Check sheet for the modelled part. Datum: model origin and axes. Units: mm. Round coordinates to 2 decimals unless told otherwise and drop trailing zeros. Loops run counter-clockwise (first coordinate to the right, second up) from the corner with the lowest first, then second, coordinate; pieces in that order, holes last. Notation, with made-up numbers: (-0.75, 5) - (40.25, 5) arc R29 cw to (40.25, 42) - close; hole circle Ø6 at (42.5, 43.25). An arc over 180 degrees is marked (long way). Put each result on its own line as item: value. Start each with the question number.
Item 1: Section check D-D, the plane x = 32. Record the cut outline in (y, z), and give its area (3 significant figures).
Item 2: Section check B-B, the plane y = 12.2. Record the cut outline in (x, z).
Item 3: Draft check along X on faces 1 (the flat face through (1, 10, -1)), 2 (the cylindrical face through (-0.1, 11.52, -13.24)). Enter one of: pulls with the +X half, pulls with the -X half, needs draft (parallel to the pull), parting line crosses it, or undercut.
Item 4: Section check C-C, the plane z = -43.5. Record the cut outline in (x, y), and give its area (3 significant figures).
Item 5: Section check A-A, the plane x = 11. Record the cut outline in (y, z).
Item 6: Gauge pin test, flat ends, axial feed: pin 1 Ø1 at (x, y) = (-33.5, 11.5) entering from +Z; pin 2 Ø0.9 at (y, z) = (12, -78.5) entering from +X; pin 3 Ø1.5 at (x, y) = (-58, 11.5) entering from -Z. Record the tip position at first contact, or that the pin passes through.
Item 7: Material ranges on line 1 along X through (y, z) = (12, 35); line 2 along Z through (x, y) = (-33.5, 12.1); line 3 along X through (y, z) = (10.5, -9.5), recorded low to high.
Autodesk Inventor part; units mm, degrees
ref_plane "YZ Plane" through (0, 0, 0) normal (1, 0, 0) x (0, 1, 0)
ref_plane "XZ Plane" through (0, 0, 0) normal (0, 1, 0) x (-1, 0, 0)
ref_plane "XY Plane" through (0, 0, 0) normal (0, 0, 1) x (1, 0, 0)
sketch "스케치1" plane through (0, 0, 0) normal (0, 1, 0) x (-1, 0, 0)
  line L0 (60, 80) -> (-60, 80)
  line L1 (-60, 80) -> (-60, -80)
  line L2 (-60, -80) -> (60, -80)
  line L3 (60, -80) -> (60, 80)
  line L4 (60, 80) -> (-60, -80) construction
  line L5 (-60, 80) -> (60, -80) construction
  point P0 (0, 0)
  dimension "d0" = 120
  dimension "d1" = 160
extrude "돌출1" add sketch "스케치1" along normal blind 60
sketch "스케치2" plane through (0, 60, 0) normal (0, 1, 0) x (1, 0, 0)
  line L0 (60, -80) -> (60, 80)
  line L1 (60, 80) -> (-60, 80)
  line L2 (55, 102.1646) -> (-55, 102.1646)
  line L3 (-55, 102.1646) -> (-55, -89.711)
  line L4 (-55, -89.711) -> (55, -89.711)
  line L5 (55, -89.711) -> (55, 102.1646)
  line L6 (-60, 80) -> (-60, -80)
  point P0 (0, 0)
  point P1 (55, 80)
  point P2 (-55, 80)
  dimension "d6" = 5
  dimension "d7" = 5
extrude "돌출2" cut sketch "스케치2" against normal blind 40 contours L5 L4 L3 L1
sketch "스케치12" plane through (60, 0, -80) normal (0, 0, -1) x (-1, 0, 0)
  line L0 (-34.8463, 10) -> (156.2634, 10)
  line L1 (156.2634, 10) -> (156.2634, -36.9465)
  line L2 (156.2634, -36.9465) -> (-34.8463, -36.9465)
  line L3 (-34.8463, -36.9465) -> (-34.8463, 10)
  line L4 (0, 0) -> (120, 0)
  point P0 (60, 0)
  dimension "d85" = 10
extrude "돌출10" cut sketch "스케치12" against normal through all
sketch "스케치13" plane through (-55, 20, 80) normal (0, 0, 1) x (1, 0, 0)
  line L0 (0, 40) -> (0, 0)
  line L1 (0, 0) -> (110, 0)
  line L2 (0, 40) -> (110, 40)
  line L3 (110, 40) -> (110, 0)
  line L4 (110, 0) -> (0, 0)
  line L5 (0, 0) -> (0, 40)
  point P0 (55, -20)
extrude "돌출11" add sketch "스케치13" against normal blind 5
sketch "스케치14" plane through (55, 20, -80) normal (0, 0, -1) x (-1, 0, 0)
  line L0 (0, 0) -> (0, 40)
  line L1 (110, 0) -> (0, 0)
  line L2 (0, 40) -> (110, 40)
  line L3 (110, 40) -> (110, 0)
  line L4 (110, 0) -> (0, 0)
  line L5 (0, 0) -> (0, 40)
  point P0 (55, -20)
extrude "돌출12" add sketch "스케치14" against normal blind 5
sketch "스케치15" plane through (60, 60, -80) normal (0, 0, -1) x (-1, 0, 0)
  point P0 (60, -60)
sketch "스케치16" plane through (60, 60, -80) normal (0, 0, -1) x (-1, 0, 0)
  point P0 (60, -60)
sketch "스케치21" plane through (0, 20, 0) normal (0, 1, 0) x (1, 0, 0)
  circle A0 centre (5.4243, 8.1678) radius 7.5
  line L0 (-49.3888, 17.2731) -> (-9.3888, 17.2731)
  line L1 (-9.3888, 17.2731) -> (-9.3888, 67.2731)
  line L2 (-9.3888, 67.2731) -> (-49.3888, 67.2731)
  line L3 (-49.3888, 67.2731) -> (-49.3888, 17.2731)
  point P0 (0, 0)
  dimension "d117" = 15
  dimension "d118" = 50
  dimension "d119" = 40
extrude "돌출15" cut sketch "스케치21" against normal through all contours A0
sketch "스케치24" plane through (0, 60, 0) normal (0, 1, 0) x (1, 0, 0)
  line L0 (-60, 80) -> (-60, -80)
  line L1 (60, 80) -> (-60, 80)
  line L2 (-60, -80) -> (60, -80)
  line L3 (60, -80) -> (60, 80)
  line L4 (60, 80) -> (-60, 80)
  line L5 (-60, 80) -> (-60, -80)
  point P0 (0, 0)
extrude "돌출17" cut sketch "스케치24" against normal blind 40
sketch "스케치25" plane through (60, 20, -80) normal (0, 0, -1) x (-1, 0, 0)
  point P0 (60, -20)
sketch "스케치26" plane through (0, 20, 0) normal (0, 1, 0) x (1, 0, 0)
  point P0 (0, 0)
sketch "스케치27" plane through (0, 20, 0) normal (0, 1, 0) x (1, 0, 0)
  line L0 (-60, -80) -> (-60, 80)
  line L1 (60, 80) -> (60, -80)
  line L2 (-60, -80) -> (60, -80)
  line L3 (60, -80) -> (60, 80)
  line L4 (60, 80) -> (-60, 80)
  line L5 (-60, 80) -> (-60, -80)
  point P0 (0, 0)
  point P1 (60, -80)
extrude "돌출18" cut sketch "스케치27" against normal blind 7
sketch "스케치30" plane through (0, 13, 0) normal (0, 1, 0) x (1, 0, 0)
  point P0 (0, 0)
sketch "스케치31" plane through (0, 13, 0) normal (0, 1, 0) x (1, 0, 0)
  line L0 (-60, -80) -> (-60, 80)
  line L1 (60, -80) -> (-60, -80)
  line L2 (60, 80) -> (60, -80)
  line L3 (-60, 80) -> (60, 80)
  line L4 (57, 77) -> (57, -77)
  line L5 (57, -77) -> (-57, -77)
  line L6 (-57, -77) -> (-57, 77)
  line L7 (-57, 77) -> (57, 77)
  point P0 (0, 0)
  dimension "d160" = 3
extrude "돌출21" cut sketch "스케치31" against normal through all
sketch "스케치32" plane through (0, 13, 0) normal (0, 1, 0) x (1, 0, 0)
  line L0 (-15, 68.5163) -> (15, 68.5163)
  line L1 (15, 68.5163) -> (15, 80)
  line L2 (15, 80) -> (-15, 80)
  line L3 (-15, 80) -> (-15, 68.5163)
  line L4 (57, 77) -> (-57, 77)
  line L5 (-57, 77) -> (-57, -77)
  line L6 (-57, 0) -> (57, 0)
  line L7 (-15, -68.5163) -> (15, -68.5163)
  line L8 (15, -68.5163) -> (15, -80)
  line L9 (15, -80) -> (-15, -80)
  line L10 (-15, -80) -> (-15, -68.5163)
  line L11 (-57, -77) -> (57, -77)
  point P0 (0, 0)
  point P1 (-15, 77)
  point P2 (15, 77)
  point P3 (15, -77)
  point P4 (-15, -77)
  dimension "d163" = 3
  dimension "d164" = 42
  dimension "d165" = 30
extrude "돌출22" add sketch "스케치32" against normal blind 3 contours L11 L8 L9 L10 | L3 L2 L1 L4
sketch "스케치33" plane through (0, 13, 0) normal (0, 1, 0) x (1, 0, 0)
  line L0 (44.1532, -15) -> (60, -15)
  line L1 (60, -15) -> (60, 15)
  line L2 (60, 15) -> (44.1532, 15)
  line L3 (44.1532, 15) -> (44.1532, -15)
  line L4 (57, -77) -> (57, 77)
  line L5 (57, 77) -> (15, 77)
  line L6 (-57, 77) -> (-57, -77)
  line L7 (-15, 80) -> (15, 80)
  line L8 (0, 80) -> (0, -80)
  line L9 (15, -80) -> (-15, -80)
  line L10 (-44.1532, -15) -> (-60, -15)
  line L11 (-60, -15) -> (-60, 15)
  line L12 (-60, 15) -> (-44.1532, 15)
  line L13 (-44.1532, 15) -> (-44.1532, -15)
  point P0 (0, 0)
  point P1 (57, 15)
  point P2 (57, -15)
  point P3 (-57, -15)
  point P4 (-57, 15)
  dimension "d168" = 3
  dimension "d169" = 30
  dimension "d170" = 62
extrude "돌출23" add sketch "스케치33" against normal blind 3 contours L4 L2 L1 L0 | L6 L10 L11 L12
sketch "스케치34" plane through (0, 13, 0) normal (0, 1, 0) x (1, 0, 0)
  point P0 (0, 0)
sketch "스케치35" plane through (0, 13, 0) normal (0, 1, 0) x (1, 0, 0)
  point P0 (0, 0)
properties part number "본체 밑판 레이저 커터"
Check result:
1. outline: (10, -77) - (13, -77) - (13, 77) - (10, 77) - close
1. area: 462 mm²
2. outline: (-60, -15) - (-57, -15) - (-57, -77) - (-15, -77) - (-15, -80) - (15, -80) - (15, -77) - (57, -77) - (57, -15) - (60, -15) - (60, 15) - (57, 15) - (57, 77) - (15, 77) - (15, 80) - (-15, 80) - (-15, 77) - (-57, 77) - (-57, 15) - (-60, 15) - close; hole circle Ø15 at (5.42, -8.17)
3. face 1: needs draft
3. face 2: undercut
4. outline: (-57, 10) - (57, 10) - (57, 13) - (-57, 13) - close
4. area: 342 mm²
5. outline: (10, -80) - (13, -80) - (13, -13.18) - (10, -13.18) - close; (10, -3.15) - (13, -3.15) - (13, 80) - (10, 80) - close
6. pin 1: z = 77
6. pin 2: x = 15
6. pin 3: z = -15
7. line 1: -57 to 57
7. line 2: -77 to 77
7. line 3: -60 to -1.96, 12.81 to 60
